Source: CAD feature listing. Evaluate the final solid. Frame: model axes, mm. A direction names the side the tool comes from. Give positions to 0.01 mm unless a question says otherwise; leave off trailing zeros. Write each loop counter-clockwise with the first axis right and the second up, starting at its lowest first coordinate (ties: lowest second). Pieces come first, ordered by that corner, then holes. Notation, with made-up numbers: (-21, 31) -> (22, 31) arc R31 cw to (22, 68) -> close; hole circle Ø9 at (39.25, 24). An arc over 180 degrees is marked (long way). Answer as a JSON object with one key per item and string values. Group by question number.
Item 1: Section query A-A on z = 7.75. Return the cut outline in (x, y), plus the area to 3 significant figures.
Item 2: Access query for faces 1 (the face through (-3, 0.4, 6)), 2 (the face through (-3, -0.4, 6)), 3 (the face through (-2.7, 0, 3)), 4 (the face through (1.75, 0, 13)). Directions: +Z, -Z, +X, -X, +Y, -Y. A direction counts if a zero-diameter tool reaches every point of the face in a straight line with its end or side. Return the directions, or none.
Item 3: Ray query, probe 1 along X at (y, z) = (0.15, 4.75); probe 2 along X at (y, z) = (-0.1, 6.5); probe 3 along Y at (x, z) = (-2.5, 7.5). Return the intervals inside material, ascending. Write a range as from..to.
Item 4: Section query D-D on x = 2. Return the cut outline in (y, z), plus the area to 3 significant figures.
Item 5: First-contact query: pin 1 Ø2 at (x, z) = (1.5, 9) entering from -Y; pin 2 Ø0.6 at (x, z) = (3, 2.5) entering from +Y; pin 3 Ø0.6 at (y, z) = (0, 7.5) entering from -X. Flat tips, straight axial feed; report the tip coordinate or a pass-through.
from build123d import *

# Parameters (mm, degrees)
SKETCH1_W             = 0.8
SKETCH1_H             = 0.8
BOSS_EXTRUDE1_DEPTH   = 13.6
SKETCH2_R             = 0.05
BOSS_EXTRUDE2_DEPTH   = 1
SKETCH3_W             = 3.5
SKETCH3_H             = 1.1
SKETCH3_W_2           = 0.8
SKETCH3_H_2           = 0.8
BOSS_EXTRUDE3_DEPTH   = 2
SKETCH6_W             = 0.8
SKETCH6_H             = 0.8
BOSS_EXTRUDE4_DEPTH   = 5
BOSS_EXTRUDE4_2_DEPTH = 5
SKETCH8_R             = 0.05
BOSS_EXTRUDE5_DEPTH   = 1
SKETCH9_R             = 0.05
BOSS_EXTRUDE6_DEPTH   = 1
LOFT1_START           = -0.4
LOFT1_DEPTH           = 0.8
LOFT2_START           = -0.4
LOFT2_DEPTH           = 0.8
FILLET1_R             = 0.4


# Read off the part's stored shape, not the designer's step: Loft1, Loft2
with BuildPart() as part:
    # Sketch1 → Boss-Extrude1 (new body)
    with BuildSketch(Plane.XY):
        Rectangle(SKETCH1_W, SKETCH1_H)
    extrude(amount=BOSS_EXTRUDE1_DEPTH)

    # Sketch2 → Boss-Extrude2 (add)
    with BuildSketch(Plane(origin=(0.4, 0, 0), x_dir=(0, 0, -1), z_dir=(1, 0, 0))):
        with Locations(Location((-0.2, -0.2, 0), (0, 0, 90))):
            Circle(SKETCH2_R)
    extrude(amount=-BOSS_EXTRUDE2_DEPTH)

    # Sketch3 → Boss-Extrude3 (add)
    # profile 1 of 3: a face of its own
    with BuildSketch(Plane.XY.offset(13.6)):
        Rectangle(SKETCH3_W, SKETCH3_H)
        Rectangle(SKETCH3_W_2, SKETCH3_H_2, mode=Mode.SUBTRACT)
    # profile 2 of 3: a face of its own
    with BuildSketch(Plane.XY.offset(13.6)):
        Rectangle(SKETCH3_W_2, SKETCH3_H_2)
    # profile 3 of 3: a face of its own
    with BuildSketch(Plane.XY.offset(13.6)):
        Rectangle(SKETCH3_W_2, SKETCH3_H_2)
    extrude(amount=-BOSS_EXTRUDE3_DEPTH)



with BuildPart() as body_2:
    # Sketch6 → Boss-Extrude4 (new body)
    with BuildSketch(Plane.XY):
        with Locations((3.1, 0)):
            Rectangle(SKETCH6_W, SKETCH6_H)
    extrude(amount=BOSS_EXTRUDE4_DEPTH)

    # Sketch8 → Boss-Extrude5 (add)
    with BuildSketch(Plane(origin=(3.5, 0, 0), x_dir=(0, 0, -1), z_dir=(1, 0, 0))):
        with Locations(Location((-0.2, -0.2, 0), (0, 0, 90))):
            Circle(SKETCH8_R)
    extrude(amount=-BOSS_EXTRUDE5_DEPTH)


with BuildPart() as body_3:
    # Sketch6 → Boss-Extrude4 2 (new body)
    with BuildSketch(Plane.XY):
        with Locations((-3.1, 0)):
            Rectangle(SKETCH6_W, SKETCH6_H)
    extrude(amount=BOSS_EXTRUDE4_2_DEPTH)

    # Sketch9 → Boss-Extrude6 (add)
    with BuildSketch(Plane(origin=(-2.7, 0, 0), x_dir=(0, 0, -1), z_dir=(1, 0, 0))):
        with Locations((-0.2, -0.2)):
            Circle(SKETCH9_R)
    extrude(amount=-BOSS_EXTRUDE6_DEPTH)


with BuildPart() as part_1:
    add(part.part)

    add(body_2.part)  # Loft1 merges body 2
    # Loft1 outline → Loft1 (add)
    with BuildSketch(Plane(origin=(0, 0, 0), x_dir=(1, 0, 0), z_dir=(0, 1.0, 2.05342141911779e-12)).offset(LOFT1_START)):
        Polygon((0.7, -11.6), (1.5, -11.6), (3.5, -5), (2.7, -5), align=None)
    extrude(amount=LOFT1_DEPTH)


    add(body_3.part)  # Loft2 merges body 3
    # Loft2 outline → Loft2 (add)
    with BuildSketch(Plane(origin=(0, 0, 0), x_dir=(1, 0, 0), z_dir=(0, 1, 0)).offset(LOFT2_START)):
        Polygon((-2.7, -5), (-3.5, -5), (-1.5, -11.6), (-0.7, -11.6), align=None)
    extrude(amount=LOFT2_DEPTH)

    # Fillet1
    fillet1_edges = [part_1.edges().sort_by_distance(p)[0] for p in [
        (-3.1, -0.4, 0),
        (-3.1, 0.4, 0),
        (3.1, -0.4, 0),
        (3.1, 0.4, 0),
        (0, -0.4, 0),
        (0, 0.4, 0),
    ]]
    fillet(fillet1_edges, radius=FILLET1_R - 0.0001)  # a hair under: the kernel refuses the full size


solid = part_1.part
Worked answers:
{
 "1": {"outline": "(-2.67, -0.4) -> (-1.87, -0.4) -> (-1.87, 0.4) -> (-2.67, 0.4) -> close; (-0.4, -0.4) -> (0.4, -0.4) -> (0.4, 0.4) -> (-0.4, 0.4) -> close; (1.87, -0.4) -> (2.67, -0.4) -> (2.67, 0.4) -> (1.87, 0.4) -> close", "area": "1.92 mm^2"},
 "2": {"face 1": "-Z, +X, -X, +Y", "face 2": "-Z, +X, -X, -Y", "face 3": "-Z, +Y, -Y", "face 4": "+Z, +X, +Y, -Y"},
 "3": {"probe 1": "-3.5..-2.7, -0.4..0.4, 2.7..3.5", "probe 2": "-3.05..-2.25, -0.4..0.4, 2.25..3.05", "probe 3": "-0.4..0.4"},
 "4": {"outline": "(-0.4, 7.31) -> (0.4, 7.31) -> (0.4, 9.95) -> (-0.4, 9.95) -> close", "area": "2.11 mm^2"},
 "5": {"pin 1": "y = -0.4", "pin 2": "y = 0.4", "pin 3": "x = -2.83"}
}
